from build123d import *

# Parameters (mm, degrees)
SKETCH1_W           = 40
SKETCH1_H           = 40
BOSS_EXTRUDE1_DEPTH = 13.413545042
SKETCH2_R           = 3
CUT_EXTRUDE1_DEPTH  = 59.13710683
SKETCH3_W           = 40
SKETCH3_H           = 73.413545042
BOSS_EXTRUDE2_DEPTH = 23.804241557
SKETCH4_R           = 1.7
CUT_EXTRUDE2_DEPTH  = 93.679817629
SKETCH5_R           = 1.7
CUT_EXTRUDE3_DEPTH  = 83.462112512
SKETCH6_R           = 16.35
SKETCH6_R_2         = 13.85
BOSS_EXTRUDE3_DEPTH = 2
BOSS_EXTRUDE4_DEPTH = 4
BOSS_EXTRUDE5_DEPTH = 4
SKETCH9_R           = 9
CUT_EXTRUDE4_DEPTH  = 2


with BuildPart() as part:
    # Sketch1 → Boss-Extrude1 (new body)
    with BuildSketch(Plane(origin=(0, 0, 0), x_dir=(1, 0, 0), z_dir=(0, 1, 0))):
        with Locations((20, 20)):
            Rectangle(SKETCH1_W, SKETCH1_H)
    extrude(amount=BOSS_EXTRUDE1_DEPTH)

    # Sketch2 → Cut-Extrude1 (cut, through all)
    with BuildSketch(Plane(origin=(0, 13.413545042, 0), x_dir=(1, 0, 0), z_dir=(0, 1, 0))):
        with Locations(Location((20, 20, 0), (0, 0, 270))):
            Circle(SKETCH2_R)
    extrude(amount=-CUT_EXTRUDE1_DEPTH, mode=Mode.SUBTRACT)

    # Sketch3 → Boss-Extrude2 (add)
    with BuildSketch(Plane.ZY):
        with Locations((-20, 36.706772521)):
            Rectangle(SKETCH3_W, SKETCH3_H)
    extrude(amount=BOSS_EXTRUDE2_DEPTH)

    # Sketch4 → Cut-Extrude2 (cut, through all)
    with BuildSketch(Plane(origin=(0, 0, 0), x_dir=(0, 0, -1), z_dir=(1, 0, 0))):
        with Locations((10, 65.131260141)):
            Circle(SKETCH4_R)
        with Locations((30, 65.131260141)):
            Circle(SKETCH4_R)
        with Locations((10, 45.131260141)):
            Circle(SKETCH4_R)
        with Locations((30, 45.131260141)):
            Circle(SKETCH4_R)
        with Locations((10, 25.131260141)):
            Circle(SKETCH4_R)
        with Locations((30, 25.131260141)):
            Circle(SKETCH4_R)
    extrude(amount=-CUT_EXTRUDE2_DEPTH, mode=Mode.SUBTRACT)

    # Sketch5 → Cut-Extrude3 (cut, through all)
    with BuildSketch(Plane(origin=(0, 13.413545042, 0), x_dir=(1, 0, 0), z_dir=(0, 1, 0))):
        with Locations(Location((20, 31, 0), (0, 0, 270))):
            Circle(SKETCH5_R)
        with Locations(Location((31, 20, 0), (0, 0, 270))):
            Circle(SKETCH5_R)
        with Locations(Location((20, 9, 0), (0, 0, 270))):
            Circle(SKETCH5_R)
        with Locations(Location((9, 20, 0), (0, 0, 270))):
            Circle(SKETCH5_R)
    extrude(amount=-CUT_EXTRUDE3_DEPTH, mode=Mode.SUBTRACT)

    # Sketch6 → Boss-Extrude3 (add)
    with BuildSketch(Plane(origin=(0, 13.413545042, 0), x_dir=(1, 0, 0), z_dir=(0, 1, 0))):
        with Locations(Location((20, 20, 0), (0, 0, 90))):
            Circle(SKETCH6_R)
        with Locations(Location((20, 20, 0), (0, 0, 270))):
            Circle(SKETCH6_R_2, mode=Mode.SUBTRACT)
    extrude(amount=BOSS_EXTRUDE3_DEPTH)

    # Sketch7 → Boss-Extrude4 (add)
    with BuildSketch(Plane(origin=(0, 0, -40), x_dir=(-1, 0, 0), z_dir=(0, 0, -1))):
        Polygon((-15, 13.413545042), (0, 28.413545042), (0, 13.413545042), align=None)
    extrude(amount=-BOSS_EXTRUDE4_DEPTH)

    # Sketch8 → Boss-Extrude5 (add)
    with BuildSketch(Plane.XY):
        Polygon((0, 28.413545042), (0, 13.413545042), (15, 13.413545042), align=None)
    extrude(amount=-BOSS_EXTRUDE5_DEPTH)

    # Sketch9 → Cut-Extrude4 (cut)
    with BuildSketch(Plane(origin=(0, 13.413545042, 0), x_dir=(1, 0, 0), z_dir=(0, 1, 0))):
        with Locations(Location((20, 20, 0), (0, 0, 270))):
            Circle(SKETCH9_R)
    extrude(amount=-CUT_EXTRUDE4_DEPTH, mode=Mode.SUBTRACT)


solid = part.part
Geometry check sheet. Reference: the model listing, model coordinates, mm. A direction names the side the tool comes from. Round coordinates to 2 decimals unless told otherwise and drop trailing zeros. Order: outer loops, then holes, each group sorted by start corner. A loop starts at its lowest first (then second) coordinate and runs counter-clockwise, first axis right, second up. Notation, with made-up numbers: M -12.5,-38.5 L 43.5,-38.5 A14 cw 43.5,-23.5 Z; hole C -2.75,-37.5 d10. An arc over 180 degrees is marked long. Answer in a Markdown table with one row per item. Add a question column.
Item 1: Draft check along X on faces 3 (the face through (8.35, 6.8, -18.43)), 4 (the face through (-12, 73.414, -20)), 5 (the face through (-23.804, 37, -20)). Enter one of: released by +X, released by -X, zero draft, split by the parting line, or undercut.
Item 2: Sectioned sample at A-A, the plane x = 20. Enter the section's corners in (y, z), plus the area to 3 significant figures.
Item 3: Sectioned sample at C-C, the plane z = -13. Enter the section's corners in (x, y).
Item 4: Sectioned sample at D-D, the plane y = 48. Enter the section's corners in (x, z).
Item 5: Material ranges on L1, parallel to Y at x = -6, z = -10; L2, parallel to X at y = 15, z = -20; L3, parallel to X at y = 5, z = -20, recorded low to high. Write a range as [from, to].
Item 6: Depth check by flat-ended pin: pin 1 Ø3 at (y, z) = (25.13, -10) entering from -X; pin 2 Ø10 at (x, z) = (26.5, -23) entering from +Y; pin 3 Ø4.5 at (y, z) = (65.13, -10) entering from +X; pin 4 Ø20 at (x, z) = (25.5, -13) entering from +Y. Enter the tip coordinate at first touch or a pass-through.
Item 7: Sectioned sample at B-B, the plane x = 31. Enter the section's corners in (y, z).
Item 8: Set-up check for faces 1 (the face through (4, 18, -4)), 2 (the face through (18.2, 5.8, -22.4)): record each of +Z, -Z, +X, -X, +Y, -Y from which the full face is reachable in a straight line by a thin tool's end or side.
Filled in:
| question | item | result |
|---|---|---|
| 1 | face 3 | undercut |
| 1 | face 4 | zero draft |
| 1 | face 5 | released by -X |
| 2 | outline | M 0,-40 L 13.41,-40 L 13.41,-36.35 L 15.41,-36.35 L 15.41,-33.85 L 13.41,-33.85 L 13.41,-32.7 L 0,-32.7 Z; M 0,-29.3 L 13.41,-29.3 L 13.41,-29 L 11.41,-29 L 11.41,-23 L 0,-23 Z; M 0,-17 L 11.41,-17 L 11.41,-11 L 13.41,-11 L 13.41,-10.7 L 0,-10.7 Z; M 0,-7.3 L 13.41,-7.3 L 13.41,-6.15 L 15.41,-6.15 L 15.41,-3.65 L 13.41,-3.65 L 13.41,0 L 0,0 Z |
| 2 | area | 351 mm² |
| 3 | outline | M -23.8,0 L 40,0 L 40,13.41 L 34.78,13.41 L 34.78,15.41 L 31.95,15.41 L 31.95,13.41 L 25.66,13.41 L 25.66,11.41 L 14.34,11.41 L 14.34,13.41 L 8.05,13.41 L 8.05,15.41 L 5.22,15.41 L 5.22,13.41 L 0,13.41 L 0,73.41 L -23.8,73.41 Z |
| 4 | outline | M -23.8,-40 L 0,-40 L 0,0 L -23.8,0 Z |
| 5 | L1 | y = [0, 23.43], [26.83, 43.43], [46.83, 63.43], [66.83, 73.41] |
| 5 | L2 | x = [-23.8, 0], [3.65, 6.15], [33.85, 36.35] |
| 5 | L3 | x = [-23.8, 7.3], [10.7, 17], [23, 29.3], [32.7, 40] |
| 6 | pin 1 | passes through |
| 6 | pin 2 | stops at y = 13.41 |
| 6 | pin 3 | stops at x = 0 |
| 6 | pin 4 | stops at y = 15.41 |
| 7 | outline | M 0,-40 L 13.41,-40 L 13.41,-32.1 L 15.41,-32.1 L 15.41,-28.42 L 13.41,-28.42 L 13.41,-21.7 L 0,-21.7 Z; M 0,-18.3 L 13.41,-18.3 L 13.41,-11.58 L 15.41,-11.58 L 15.41,-7.9 L 13.41,-7.9 L 13.41,0 L 0,0 Z |
| 8 | face 1 | +Y |
| 8 | face 2 | +Y, -Y |
